```python
from build123d import *

# Parameters (mm, degrees)
BOSS_EXTRUDE1_DEPTH      = 2
BOSS_EXTRUDE1_DEPTH_BACK = 2
SKETCH3_R                = 1.75
CUT_EXTRUDE2_DEPTH       = 80.221209281


with BuildPart() as part:
    # Sketch3 → Boss-Extrude1 (new, two sides: drawn at the far end of the back side and taken through both)
    with BuildSketch(Plane.XY.offset(-BOSS_EXTRUDE1_DEPTH_BACK)):
        with BuildLine():
            Line((-11.440860215, -54.818853669), (-9.985215054, -47.844133447))
            Line((-9.985215054, -47.844133447), (-23.069216943, -43.342064897))
            ThreePointArc((-23.069216943, -43.342064897), (-25.874137738, -43.964725959), (-28.586767, -43.017662099))
            ThreePointArc((-28.586767, -43.017662099), (0, 47.3), (28.586767, -43.017662099))
            ThreePointArc((28.586767, -43.017662099), (25.874137738, -43.964725959), (23.069216943, -43.342064897))
            Line((23.069216943, -43.342064897), (9.985215054, -47.844133447))
            Line((9.985215054, -47.844133447), (11.440860215, -54.818853669))
            ThreePointArc((11.440860215, -54.818853669), (0, 56), (-11.440860215, -54.818853669))
        make_face()
        with Locations((-16.631028749, -48.333429201)):
            Circle(SKETCH3_R, mode=Mode.SUBTRACT)
        with Locations(Location((16.631028749, -48.333429201, 0), (0, 0, 180))):
            Circle(SKETCH3_R, mode=Mode.SUBTRACT)
    extrude(amount=BOSS_EXTRUDE1_DEPTH + BOSS_EXTRUDE1_DEPTH_BACK)

    # Sketch5 → Cut-Extrude2 (cut, symmetric)
    with BuildSketch(Plane.XY):
        with BuildLine():
            Line((-23.069216943, -43.342064897), (0, 0))
            Line((0, 0), (-9.985215054, -47.844133447))
            ThreePointArc((-9.985215054, -47.844133447), (-16.608557726, -45.829496133), (-23.069216943, -43.342064897))
        make_face()
    cut_extrude2 = extrude(amount=CUT_EXTRUDE2_DEPTH, both=True, mode=Mode.SUBTRACT)

    # Mirror1: Cut-Extrude2 across plane
    add(cut_extrude2.mirror(Plane(origin=(0, 0, 0), x_dir=(0, 0, 1), z_dir=(1, 0, 0))), mode=Mode.SUBTRACT)


solid = part.part
```
Here's how the part is built. I have some questions about the finished solid (model axes, mm). A direction names the side the tool comes from. Round coordinates to 2 decimals unless told otherwise and drop trailing zeros. Write each loop counter-clockwise with the first axis right and the second up, starting at its lowest first coordinate (ties: lowest second). Pieces come first, ordered by that corner, then holes.
Q1. Will these pins go through, and if not, where does the flat tip stop? P1, Ø2, axis at x = -16.63, y = -48.33, coming from the +Z side; P2, Ø1.5, axis at y = -11.5, z = 0, coming from the -X side; P3, Ø1, axis at y = 14.5, z = 0.5, coming from the +X side; P4, Ø2, axis at x = 41.5, z = -1.5, coming from the +Y side.
Q2. Which directions (+Z, -Z, +X, -X, +Y, -Y) give clear straight access to the entire face, cutting with the end or side of a thin tool? Please do faces 1 (the flat face through (10.703, -51.283, -0.028)), 2 (the cylindrical face through (-16.52, -45.86, 0.03)), 3 (the flat face through (12, 46, -2)).
Q3. If we mould it in two halves opening along X, with no side actions, what happens to faces 4 (the flat face through (12, 46, 2)), 5 (the cylindrical face through (2.301, 55.953, -0.028)), 6 (the flat face through (-10.723, -51.38, -0.028))? For each: +X half, -X half, draft (parallel to the pull), parting line (faces both ways), or undercut.
Q4. If we section it at A-A on x = -25: Write out the boundary of the cut face in (y, z).
Q5. If we section it at C-C on z = 1.35: Write out the boundary of the cut face in (x, y), plus the area to 3 significant figures.
Q6. If we section it at B-B on y = 17.5: Write out the boundary of the cut face in (x, z).
Q7. Please list where these lines run through material, in increasing order: probe 1 along X at (y, z) = (-1, 0.75); probe 2 along X at (y, z) = (-49, 1.2); probe 3 along X at (y, z) = (-12, -1.2).
Q8. If we section it at D-D on x = 0: Write out the boundary of the cut face in (y, z).
Answer below:
1. P1: passes through
1. P2: stops at x = -54.96
1. P3: stops at x = 54.22
1. P4: stops at y = 38.67
2. face 1: +Z, -Z, -Y
2. face 2: +Z, -Z
2. face 3: -Z, +X, -X, +Y, -Y
3. face 4: draft
3. face 5: parting line
3. face 6: undercut
4. outline: (-50.11, -2) - (-43.94, -2) - (-43.94, 2) - (-50.11, 2) - close; (40.55, -2) - (50.11, -2) - (50.11, 2) - (40.55, 2) - close
5. outline: (-28.59, -43.02) arc R49.68 cw (long way) to (28.59, -43.02) arc R5.25 cw to (23.07, -43.34) arc R95.85 cw to (9.99, -47.84) - (11.44, -54.82) arc R56 ccw (long way) to (-11.44, -54.82) - (-9.99, -47.84) arc R95.85 cw to (-23.07, -43.34) arc R5.25 cw to start; hole circle Ø3.5 at (-16.63, -48.33); hole circle Ø3.5 at (16.63, -48.33)
5. area: 2,090 mm2
6. outline: (-53.2, -2) - (-45.53, -2) - (-45.53, 2) - (-53.2, 2) - close; (45.53, -2) - (53.2, -2) - (53.2, 2) - (45.53, 2) - close
7. probe 1: x = -55.99 to -49.66, 49.66 to 55.99
7. probe 2: x = -27.11 to -18.25, -15.01 to -10.23, 10.23 to 15.01, 18.25 to 27.11
7. probe 3: x = -54.7 to -48.74, 48.74 to 54.7
8. outline: (47.3, -2) - (56, -2) - (56, 2) - (47.3, 2) - close
